from build123d import *

# Parameters (mm, degrees)
F0_R     = 101.6
F1_DEPTH = 101.6
F3_R     = 25.4
F4_DEPTH = 76.2
F6_R     = 25.4
F7_DEPTH = 76.2


with BuildPart() as f1:
    # F0 (on Front) → F1 (new body)
    with BuildSketch(Plane.XZ):
        Circle(F0_R)
    extrude(amount=F1_DEPTH)

    # F3 (on offset) → F4 (cut)
    with BuildSketch(Plane.XY.offset(101.6)):
        with Locations((0, -50.8)):
            Circle(F3_R)
    extrude(amount=-F4_DEPTH, mode=Mode.SUBTRACT)

    # F6 (on offset) → F7 (cut)
    with BuildSketch(Plane.XY.offset(-101.6)):
        with Locations((0, -50.8)):
            Circle(F6_R)
    extrude(amount=F7_DEPTH, mode=Mode.SUBTRACT)


solid = f1.part
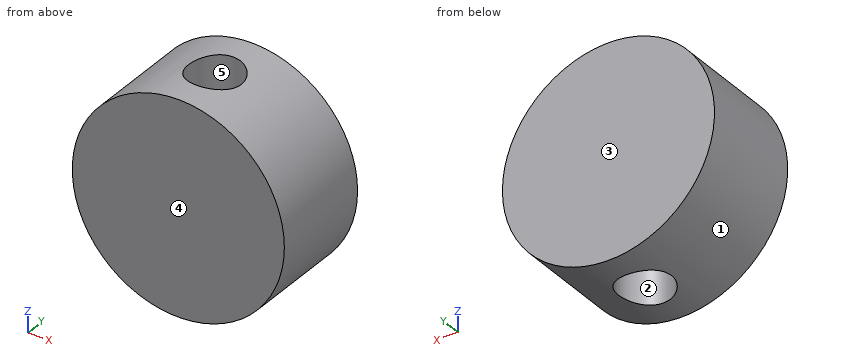
Can you work these out from the model? Positions are in its coordinate system, mm. Face numbers are marked on the shaded views. A direction names the side the tool comes from. Round coordinates to 2 decimals unless told otherwise and drop trailing zeros. Write each loop counter-clockwise with the first axis right and the second up, starting at its lowest first coordinate (ties: lowest second). Pieces come first, ordered by that corner, then holes. Notation, with made-up numbers: M 12,79.5 L 46,79.5 A27 ccw 46,106.5 Z; hole C 62,6 d8. An arc over 180 degrees is marked long. Use a Markdown table: item, result.
Item 1: I want a section at D-D (z = 72.5). List the corners of the cut face in (x, y) for me, and give its area (3 significant figures).
Found:
| item | result |
|---|---|
| outline | M -71.18,-101.6 L 71.18,-101.6 L 71.18,0 L -71.18,0 Z; hole C 0,-50.8 d50.8 |
| area | 12,400 mm2 |
Item 2: If I drill on line 1 along Y through (x, z) = (0, -69); line 2 along X through (y, z) = (-50.8, -67); line 3 along X through (y, z) = (-22, 0.5), over which ranges is the centre line in solid material (lowest first)? Write a range as [from, to].
Found:
| item | result |
|---|---|
| line 1 | y = [-101.6, -76.2], [-25.4, 0] |
| line 2 | x = [-76.38, -25.4], [25.4, 76.38] |
| line 3 | x = [-101.6, 101.6] |
Item 3: Which directions (+Z, -Z, +X, -X, +Y, -Y) give clear straight access to the entire face, cutting with the end or side of a thin tool? Please do the marked faces 4 and 5.
Found:
| item | result |
|---|---|
| face 4 | +Z, -Z, +X, -X, -Y |
| face 5 | +Z |
Item 4: For pin 1 Ø1.5 at (y, z) = (-43.5, 41.5) entering from -X; pin 2 Ø5 at (x, y) = (26, -18.5) entering from -Z; pin 3 Ø4 at (x, y) = (-61.5, -29) entering from +Z, each with a flat end and sliding along its axis, tell me the tip position at first contact or that it passes through.
Found:
| item | result |
|---|---|
| pin 1 | stops at x = -93.07 |
| pin 2 | stops at z = -98.84 |
| pin 3 | stops at z = 82.35 |
Item 5: I want a section at B-B (x = 0). List the corners of the cut face in (y, z) for me, and give its area (3 significant figures).
Found:
| item | result |
|---|---|
| outline | M -101.6,-101.6 L -76.2,-101.6 L -76.2,-25.4 L -25.4,-25.4 L -25.4,-101.6 L 0,-101.6 L 0,101.6 L -25.4,101.6 L -25.4,25.4 L -76.2,25.4 L -76.2,101.6 L -101.6,101.6 Z |
| area | 12,900 mm2 |
Item 6: I want a section at A-A (z = 49). List the corners of the cut face in (x, y) for me.
Found:
| item | result |
|---|---|
| outline | M -89,-101.6 L 89,-101.6 L 89,0 L -89,0 Z; hole C 0,-50.8 d50.8 |
Item 7: We'd pull the mould along X, two halves only. Please class the marked faces 1, 2 and 3: released by +X, released by -X, zero draft, split by the parting line, or undercut.
Found:
| item | result |
|---|---|
| face 1 | split by the parting line |
| face 2 | undercut |
| face 3 | zero draft |
Item 8: I want a section at C-C (y = -18). List the corners of the cut face in (x, z) for me, and give its area (3 significant figures).
Found:
| item | result |
|---|---|
| outline | C 0,0 d203.2 |
| area | 32,400 mm2 |
